```python
from build123d import *

# Parameters (mm, degrees)
SKETCH_1_R      = 3.45
EXTRUDE_1_DEPTH = 2.5
FILLET_1_R      = 2


with BuildPart() as part:
    # 草图1 → 凸台-拉伸1 (new body)
    with BuildSketch(Plane(origin=(0, 0, 0), x_dir=(1, 0, 0), z_dir=(0, 1, 0))):
        Polygon((13, -13), (42.5, -13), (42.5, 13), (-42.5, 13), (-42.5, -13), (-13, -13), (-13, -72), (13, -72), align=None)
        with Locations((0, -60)):
            Circle(SKETCH_1_R, mode=Mode.SUBTRACT)
        with Locations((0, -30)):
            Circle(SKETCH_1_R, mode=Mode.SUBTRACT)
        with Locations((-30.5, 0)):
            Circle(SKETCH_1_R, mode=Mode.SUBTRACT)
        with Locations((30.5, 0)):
            Circle(SKETCH_1_R, mode=Mode.SUBTRACT)
    extrude(amount=EXTRUDE_1_DEPTH)

    # 圆角1
    fillet_1_edges = [part.edges().sort_by_distance(p)[0] for p in [
        (42.5, 1.25, 13),
        (13, 1.25, 13),
        (13, 1.25, 72),
        (-13, 1.25, 72),
        (-13, 1.25, 13),
        (-42.5, 1.25, 13),
        (-42.5, 1.25, -13),
        (42.5, 1.25, -13),
    ]]
    fillet(fillet_1_edges, radius=FILLET_1_R)


solid = part.part
```
The model under review builds one solid part; all positions refer to its coordinate system, in mm. A direction names the side the tool comes from. Coordinates: 2 decimals unless noted, no trailing zeros. Write each loop counter-clockwise with the first axis right and the second up, starting at its lowest first coordinate (ties: lowest second). Pieces come first, ordered by that corner, then holes. Notation, with made-up numbers: (26.25, 84) - (83.25, 84) arc R25 ccw to (83.25, 111) - close; hole circle Ø3 at (84, 3). An arc over 180 degrees is marked (long way). Answer in a Markdown table with one row per item. Add a question column.
Q1. To check wall thickness, follow line 1 along X through (y, z) = (0.7, 0); line 2 along Z through (x, y) = (0, 0.95); line 3 along Z through (x, y) = (30.5, 1.05). State the ranges of each line that lie inside material, in increasing order. Write a range as from..to.
Q2. Consider section B-B on y = 2.05. Give the boundary of the cut face in (x, z).
Q3. Consider section A-A on x = 0. Give the boundary of the cut face in (y, z), then the cut area to 3 significant figures.
Q4. Draft analysis for pull direction X (two halves, no side actions). For faces 3 (the face through (-42.5, 1, 0)), 4 (the face through (-33.947, 1.232, -0.152)), 5 (the face through (13, 1, 43)), state which applies: +X half, -X half, draft (parallel to the pull), parting line (faces both ways), or undercut.
Q5. For faces 1 (the face through (-0.748, 1.232, 33.368)), 2 (the face through (-28, 1, 13)), list the 3-axis set-ups (+Z, -Z, +X, -X, +Y, -Y) from which the entire face can be reached by the end or side of a thin tool; tool diameter is ignored.
Q6. Clearance check with a flat-ended pin moving along its axis: pin 1 (1.2 mm diameter, centred on y = 1.5, z = 49.5, fed in from -X). State where the tip first meets the part, or that it passes through.
Q7. Consider section C-C on z = 0. Give the boundary of the cut face in (x, y), then the cut area to 3 significant figures.
Q8. Consider section D-D on x = -30.5. Give the boundary of the cut face in (y, z).
Answers below:
| question | item | result |
|---|---|---|
| 1 | line 1 | -42.5..-33.95, -27.05..27.05, 33.95..42.5 |
| 1 | line 2 | -13..26.55, 33.45..56.55, 63.45..72 |
| 1 | line 3 | -13..-3.45, 3.45..13 |
| 2 | outline | (-42.5, -11) arc R2 ccw to (-40.5, -13) - (40.5, -13) arc R2 ccw to (42.5, -11) - (42.5, 11) arc R2 ccw to (40.5, 13) - (15, 13) arc R2 cw to (13, 15) - (13, 70) arc R2 ccw to (11, 72) - (-11, 72) arc R2 ccw to (-13, 70) - (-13, 15) arc R2 cw to (-15, 13) - (-40.5, 13) arc R2 ccw to (-42.5, 11) - close; hole circle Ø6.9 at (-30.5, 0); hole circle Ø6.9 at (0, 30); hole circle Ø6.9 at (0, 60); hole circle Ø6.9 at (30.5, 0) |
| 3 | outline | (0, -13) - (2.5, -13) - (2.5, 26.55) - (0, 26.55) - close; (0, 33.45) - (2.5, 33.45) - (2.5, 56.55) - (0, 56.55) - close; (0, 63.45) - (2.5, 63.45) - (2.5, 72) - (0, 72) - close |
| 3 | area | 178 mm² |
| 4 | face 3 | -X half |
| 4 | face 4 | undercut |
| 4 | face 5 | +X half |
| 5 | face 1 | +Y, -Y |
| 5 | face 2 | +Z, -X, +Y, -Y |
| 6 | pin 1 | x = -13 |
| 7 | outline | (-42.5, 0) - (-33.95, 0) - (-33.95, 2.5) - (-42.5, 2.5) - close; (-27.05, 0) - (27.05, 0) - (27.05, 2.5) - (-27.05, 2.5) - close; (33.95, 0) - (42.5, 0) - (42.5, 2.5) - (33.95, 2.5) - close |
| 7 | area | 178 mm² |
| 8 | outline | (0, -13) - (2.5, -13) - (2.5, -3.45) - (0, -3.45) - close; (0, 3.45) - (2.5, 3.45) - (2.5, 13) - (0, 13) - close |
